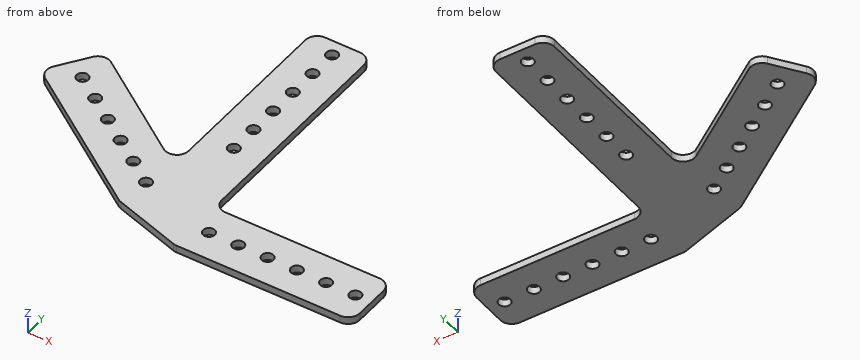
```python
from build123d import *

# Parameters (mm, degrees)
BOSS_EXTRUDE1_DEPTH     = 3.175
CUT_EXTRUDE5_START      = 3.175
SKETCH3_R               = 2.54
CUT_EXTRUDE5_DEPTH      = 4.175
CUT_EXTRUDE5_DEPTH_BACK = 4.175


with BuildPart() as part:
    # Sketch2 → Boss-Extrude1 (new body)
    with BuildSketch(Plane.XY):
        with BuildLine():
            Line((-20.32, 127.404287689), (-5.08, 127.404287689))
            ThreePointArc((-5.08, 127.404287689), (-1.487897552, 125.916390137), (0, 122.324287689))
            Line((0, 122.324287689), (0, 50.8))
            Line((0, 50.8), (0, 30.48))
            ThreePointArc((0, 30.48), (1.487897552, 26.887897552), (5.08, 25.4))
            Line((5.08, 25.4), (71.811597359, 25.4))
            ThreePointArc((71.811597359, 25.4), (75.403699807, 23.912102448), (76.891597359, 20.32))
            Line((76.891597359, 20.32), (76.891597359, 5.08))
            ThreePointArc((76.891597359, 5.08), (75.403699807, 1.487897552), (71.811597359, 0))
            Line((71.811597359, 0), (0.781886783, 0))
            ThreePointArc((0.781886783, 0), (0.009099981, 0.059123527), (-0.745698678, 0.23511789))
            Line((-0.745698678, 0.23511789), (-29.641953026, 9.346071889))
            ThreePointArc((-29.641953026, 9.346071889), (-30.36119411, 9.634840472), (-31.028135861, 10.029661614))
            Line((-31.028135861, 10.029661614), (-91.189980426, 52.155438691))
            ThreePointArc((-91.189980426, 52.155438691), (-93.279035515, 55.434598334), (-92.437504515, 59.230499373))
            Line((-92.437504515, 59.230499373), (-83.696199625, 71.714376528))
            ThreePointArc((-83.696199625, 71.714376528), (-80.417039982, 73.803431616), (-76.621138943, 72.961900616))
            Line((-76.621138943, 72.961900616), (-33.393768297, 42.693769833))
            ThreePointArc((-33.393768297, 42.693769833), (-28.134317045, 42.349047185), (-25.4, 46.855062218))
            Line((-25.4, 46.855062218), (-25.4, 122.324287689))
            ThreePointArc((-25.4, 122.324287689), (-23.912102448, 125.916390137), (-20.32, 127.404287689))
        make_face()
    extrude(amount=BOSS_EXTRUDE1_DEPTH)

    # Sketch3 → Cut-Extrude5 (cut, two sides)
    with BuildSketch(Plane.XY.offset(CUT_EXTRUDE5_START)) as cut_extrude5_sk:
        with Locations((-12.7, 57.15)):
            Circle(SKETCH3_R)
        with Locations((6.35, 12.7)):
            Circle(SKETCH3_R)
        with Locations((-28.304846444, 23.626631112)):
            Circle(SKETCH3_R)
        with Locations((-38.708077406, 30.911051854)):
            Circle(SKETCH3_R)
        with Locations((-49.111308369, 38.195472596)):
            Circle(SKETCH3_R)
        with Locations((-59.514539331, 45.479893337)):
            Circle(SKETCH3_R)
        with Locations((-69.917770294, 52.764314079)):
            Circle(SKETCH3_R)
        with Locations((-80.321001256, 60.048734821)):
            Circle(SKETCH3_R)
        with Locations((-12.7, 69.85)):
            Circle(SKETCH3_R)
        with Locations((-12.7, 82.55)):
            Circle(SKETCH3_R)
        with Locations((-12.7, 95.25)):
            Circle(SKETCH3_R)
        with Locations((-12.7, 107.95)):
            Circle(SKETCH3_R)
        with Locations((-12.7, 120.65)):
            Circle(SKETCH3_R)
        with Locations((19.05, 12.7)):
            Circle(SKETCH3_R)
        with Locations((31.75, 12.7)):
            Circle(SKETCH3_R)
        with Locations((44.45, 12.7)):
            Circle(SKETCH3_R)
        with Locations((57.15, 12.7)):
            Circle(SKETCH3_R)
        with Locations((69.85, 12.7)):
            Circle(SKETCH3_R)
    extrude(amount=CUT_EXTRUDE5_DEPTH, mode=Mode.SUBTRACT)
    extrude(cut_extrude5_sk.sketch, amount=-CUT_EXTRUDE5_DEPTH_BACK, mode=Mode.SUBTRACT)


solid = part.part
```
For this review, take the finished solid that the model builds, in its own axes (mm). Round coordinates to 2 decimals unless told otherwise and drop trailing zeros. Write each loop counter-clockwise with the first axis right and the second up, starting at its lowest first coordinate (ties: lowest second). Pieces come first, ordered by that corner, then holes. Notation, with made-up numbers: (23.5, -33) -> (63.5, -33) arc R19 cw to (63.5, -2) -> close; hole circle Ø9 at (-13, 69). An arc over 180 degrees is marked (long way). Use one line per item in the form item = value.
Q1. Consider section C-C (y = 69.85). State the section outline as (x, z) points (3 decimals), then the cut area to 3 significant figures.
Resolved:
outline = (-85.002, 0) -> (-72.177, 0) -> (-72.177, 3.175) -> (-85.002, 3.175) -> close; (-25.4, 0) -> (-15.24, 0) -> (-15.24, 3.175) -> (-25.4, 3.175) -> close; (-10.16, 0) -> (0, 0) -> (0, 3.175) -> (-10.16, 3.175) -> close
area = 105 mm²
Q2. Consider section D-D (x = 65.5). State the section outline as (y, z) points (3 decimals).
Resolved:
outline = (0, 0) -> (25.4, 0) -> (25.4, 3.175) -> (0, 3.175) -> close
Q3. Clearance check with a flat-ended pin moving along its axis: pin 1 Ø1.5 at (y, z) = (44.5, 2.5) entering from -X. State where the tip first meets the part, or that it passes through.
Resolved:
pin_1 = -81.33
Q4. Consider section A-A (y = 107.95). State the section outline as (x, z) points (3 decimals), then the cut area to 3 significant figures.
Resolved:
outline = (-25.4, 0) -> (-15.24, 0) -> (-15.24, 3.175) -> (-25.4, 3.175) -> close; (-10.16, 0) -> (0, 0) -> (0, 3.175) -> (-10.16, 3.175) -> close
area = 64.5 mm²
Q5. To check wall thickness, follow probe 1 along X at (y, z) = (44, 2.65); probe 2 along Y at (x, z) = (69.5, 3.05); probe 3 along X at (y, z) = (91.5, 1.95). State the ranges of each line that lie inside material, in increasing order. Write a range as from..to.
Resolved:
probe_1 = -79.54..-61.58, -57.45..-35.26, -26.28..0
probe_2 = 0..10.18, 15.22..25.4
probe_3 = -25.4..0
Q6. Consider section B-B (x = 31.75). State the section outline as (y, z) points (3 decimals).
Resolved:
outline = (0, 0) -> (10.16, 0) -> (10.16, 3.175) -> (0, 3.175) -> close; (15.24, 0) -> (25.4, 0) -> (25.4, 3.175) -> (15.24, 3.175) -> close
